Geometry check sheet. Reference: drawing and pictorial views, mm from the part's lowest x, y, z. A direction names the side the tool comes from. Round coordinates to 2 decimals unless told otherwise and drop trailing zeros. Loops run counter-clockwise (first coordinate to the right, second up) from the corner with the lowest first, then second, coordinate; pieces in that order, holes last. Notation, with made-up numbers: (75, 75.25) -> (89, 75.25) arc R29 ccw to (89, 97.25) -> close; hole circle Ø10 at (14.25, 89.25). An arc over 180 degrees is marked (long way). Use one line per item in the form item = value.
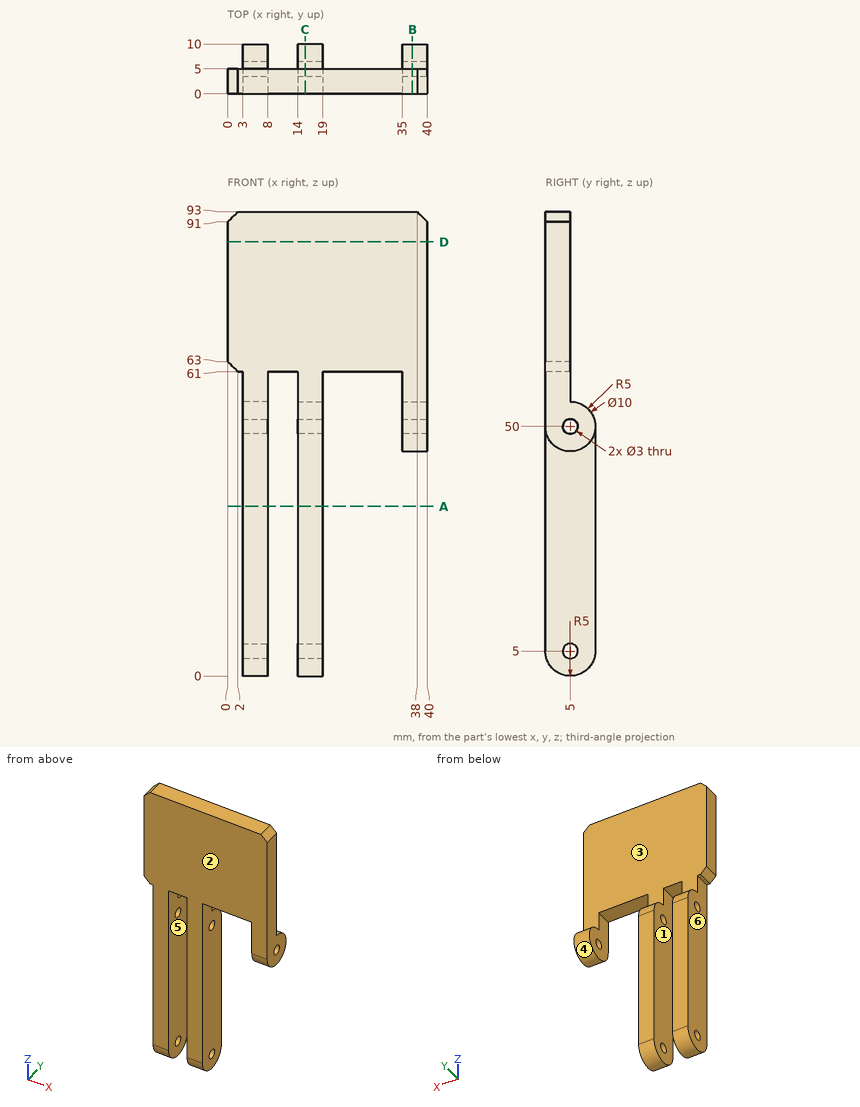
1. Tool access check on the marked faces 1, 2 and 3. Record the directions out of +Z, -Z, +X, -X, +Y, -Y that give a thin tool (end or side, any length) a straight path to the whole face; none if there is none.
Return value:
face_1 = -Z, +Y, -Y
face_2 = +Z, -Z, +X, -X, -Y
face_3 = +Z, +X, -X, +Y
2. Gauge pin test, flat ends, axial feed: pin 1 (3 mm diameter, centred on y = 5, z = 23, fed in from -X); pin 2 (3 mm diameter, centred on y = 6.5, z = 41, fed in from +X); pin 3 (2 mm diameter, centred on x = 4, z = 12.5, fed in from -Y); pin 4 (1.5 mm diameter, centred on x = 12.5, z = 66.5, fed in from +Y). Record the tip position at first contact, or that the pin passes through.
Return value:
pin_1 = 3
pin_2 = 19
pin_3 = 0
pin_4 = 5
3. Section check A-A (z = 34). Record the boundary of the cut face in (x, y), then the cut area to 3 significant figures.
Return value:
outline = (3, 0) -> (8, 0) -> (8, 10) -> (3, 10) -> close; (14, 0) -> (19, 0) -> (19, 10) -> (14, 10) -> close
area = 100 mm2
4. Mould release check, pull along X, two halves, no side actions. Record for the marked faces 4, 5 and 6: released by +X, released by -X, zero draft, split by the parting line, or undercut.
Return value:
face_4 = zero draft
face_5 = undercut
face_6 = released by -X
5. Section check D-D (z = 87). Record the boundary of the cut face in (x, y).
Return value:
outline = (0, 0) -> (40, 0) -> (40, 5) -> (0, 5) -> close
6. Material ranges on line 1 along X through (y, z) = (0.75, 55.5); line 2 along Y through (x, z) = (5.45, 50); line 3 along Z through (x, y) = (15.5, 4), recorded low to high.
Return value:
line_1 = 3 to 8, 14 to 19, 35 to 40
line_2 = 0 to 3.5, 6.5 to 10
line_3 = 0.1 to 3.88, 6.12 to 48.88, 51.12 to 93
7. Section check C-C (x = 15.5). Record the boundary of the cut face in (y, z).
Return value:
outline = (0, 5) arc R5 ccw to (10, 5) -> (10, 50) arc R5 ccw to (5, 55) -> (5, 93) -> (0, 93) -> close; hole circle Ø3 at (5, 5); hole circle Ø3 at (5, 50)
8. Section check B-B (x = 37). Record the boundary of the cut face in (y, z).
Return value:
outline = (0, 50) arc R5 ccw (long way) to (5, 55) -> (5, 93) -> (0, 93) -> close; hole circle Ø3 at (5, 50)
